```python
from build123d import *

# Parameters (mm, degrees)
SKETCH2_W           = 25
SKETCH2_H           = 62.5
SKETCH2_H_2         = 25
SKETCH2_W_2         = 62.5
BOSS_EXTRUDE3_DEPTH = 20
FILLET1_R           = 10
FILLET2_R           = 10
FILLET3_R           = 10
FILLET4_R           = 10
FILLET5_RADIUS      = 12.5
FILLET5_LENGTH      = 20
FILLET6_RADIUS      = 12.5
FILLET6_LENGTH      = 20
FILLET7_RADIUS      = 12.5
FILLET7_LENGTH      = 20
FILLET8_RADIUS      = 12.5
FILLET8_LENGTH      = 20
SKETCH4_R           = 2.5
CUT_EXTRUDE2_DEPTH  = 25
SKETCH5_R           = 37.5
BOSS_EXTRUDE4_DEPTH = 20
SKETCH7_R           = 2.5
CUT_EXTRUDE3_DEPTH  = 25
FILLET9_R           = 8


with BuildPart() as part:
    # Sketch2 → Boss-Extrude3 (new body)
    with BuildSketch(Plane(origin=(0, 0, 0), x_dir=(1, 0, 0), z_dir=(0, 1, 0))):
        with Locations((0, -43.75)):
            Rectangle(SKETCH2_W, SKETCH2_H)
        Rectangle(SKETCH2_W, SKETCH2_H_2)
        with Locations((0, 43.75)):
            Rectangle(SKETCH2_W, SKETCH2_H)
        with Locations((-43.75, 0)):
            Rectangle(SKETCH2_W_2, SKETCH2_H_2)
        with Locations((43.75, 0)):
            Rectangle(SKETCH2_W_2, SKETCH2_H_2)
    extrude(amount=BOSS_EXTRUDE3_DEPTH)

    # Fillet1
    fillet1_edges = [part.edges().sort_by_distance(p)[0] for p in [
        (-12.5, 10, 12.5),
    ]]
    fillet(fillet1_edges, radius=FILLET1_R)

    # Fillet2
    fillet2_edges = [part.edges().sort_by_distance(p)[0] for p in [
        (12.5, 10, 12.5),
    ]]
    fillet(fillet2_edges, radius=FILLET2_R)

    # Fillet3
    fillet3_edges = [part.edges().sort_by_distance(p)[0] for p in [
        (-12.5, 10, -12.5),
    ]]
    fillet(fillet3_edges, radius=FILLET3_R)

    # Fillet4
    fillet4_edges = [part.edges().sort_by_distance(p)[0] for p in [
        (12.5, 10, -12.5),
    ]]
    fillet(fillet4_edges, radius=FILLET4_R)

    # Fillet5: full round fillet: the end face becomes a half cylinder, R = half its width
    fillet5_face = Plane((75, 10, 0), x_dir=(0, 1, 0), z_dir=(1, 0, 0))  # on the end face: x along it, z out of the body
    fillet5_slab = fillet5_face.offset(-FILLET5_RADIUS / 2) * Box(FILLET5_LENGTH, 2 * FILLET5_RADIUS, FILLET5_RADIUS, mode=Mode.PRIVATE)  # the body's end, R deep
    fillet5_round = Plane((62.5, 10, 0), x_dir=(1, 0, 0), z_dir=(0, 1, 0)) * Cylinder(FILLET5_RADIUS, FILLET5_LENGTH, mode=Mode.PRIVATE)  # its axis R under the face
    add(fillet5_slab - fillet5_round, mode=Mode.SUBTRACT)

    # Fillet6: full round fillet: the end face becomes a half cylinder, R = half its width
    fillet6_face = Plane((0, 10, 75), x_dir=(0, 1, 0), z_dir=(0, 0, 1))  # on the end face: x along it, z out of the body
    fillet6_slab = fillet6_face.offset(-FILLET6_RADIUS / 2) * Box(FILLET6_LENGTH, 2 * FILLET6_RADIUS, FILLET6_RADIUS, mode=Mode.PRIVATE)  # the body's end, R deep
    fillet6_round = Plane((0, 10, 62.5), x_dir=(0, 0, 1), z_dir=(0, 1, 0)) * Cylinder(FILLET6_RADIUS, FILLET6_LENGTH, mode=Mode.PRIVATE)  # its axis R under the face
    add(fillet6_slab - fillet6_round, mode=Mode.SUBTRACT)

    # Fillet7: full round fillet: the end face becomes a half cylinder, R = half its width
    fillet7_face = Plane((-75, 10, 0), x_dir=(0, 1, 0), z_dir=(-1, 0, 0))  # on the end face: x along it, z out of the body
    fillet7_slab = fillet7_face.offset(-FILLET7_RADIUS / 2) * Box(FILLET7_LENGTH, 2 * FILLET7_RADIUS, FILLET7_RADIUS, mode=Mode.PRIVATE)  # the body's end, R deep
    fillet7_round = Plane((-62.5, 10, 0), x_dir=(-1, 0, 0), z_dir=(0, 1, 0)) * Cylinder(FILLET7_RADIUS, FILLET7_LENGTH, mode=Mode.PRIVATE)  # its axis R under the face
    add(fillet7_slab - fillet7_round, mode=Mode.SUBTRACT)

    # Fillet8: full round fillet: the end face becomes a half cylinder, R = half its width
    fillet8_face = Plane((0, 10, -75), x_dir=(0, 1, 0), z_dir=(0, 0, -1))  # on the end face: x along it, z out of the body
    fillet8_slab = fillet8_face.offset(-FILLET8_RADIUS / 2) * Box(FILLET8_LENGTH, 2 * FILLET8_RADIUS, FILLET8_RADIUS, mode=Mode.PRIVATE)  # the body's end, R deep
    fillet8_round = Plane((0, 10, -62.5), x_dir=(0, 0, -1), z_dir=(0, 1, 0)) * Cylinder(FILLET8_RADIUS, FILLET8_LENGTH, mode=Mode.PRIVATE)  # its axis R under the face
    add(fillet8_slab - fillet8_round, mode=Mode.SUBTRACT)

    # Sketch4 → Cut-Extrude2 (cut)
    with BuildSketch(Plane(origin=(0, 20, 0), x_dir=(1, 0, 0), z_dir=(0, 1, 0))):
        with Locations(Location((64, 0, 0), (0, 0, 270))):
            Circle(SKETCH4_R)
        with Locations(Location((0, -64, 0), (0, 0, 270))):
            Circle(SKETCH4_R)
        with Locations(Location((-64, 0, 0), (0, 0, 270))):
            Circle(SKETCH4_R)
        with Locations(Location((0, 64, 0), (0, 0, 270))):
            Circle(SKETCH4_R)
    extrude(amount=-CUT_EXTRUDE2_DEPTH, mode=Mode.SUBTRACT)

    # Sketch5 → Boss-Extrude4 (add)
    with BuildSketch(Plane(origin=(0, 20, 0), x_dir=(1, 0, 0), z_dir=(0, 1, 0))):
        Circle(SKETCH5_R)
    extrude(amount=-BOSS_EXTRUDE4_DEPTH)

    # Sketch7 → Cut-Extrude3 (cut)
    with BuildSketch(Plane(origin=(0, 20, 0), x_dir=(1, 0, 0), z_dir=(0, 1, 0))):
        with Locations(Location((0, 33, 0), (0, 0, 270))):
            Circle(SKETCH7_R)
        with Locations(Location((33, 0, 0), (0, 0, 270))):
            Circle(SKETCH7_R)
        with Locations(Location((0, -33, 0), (0, 0, 270))):
            Circle(SKETCH7_R)
        with Locations(Location((-33, 0, 0), (0, 0, 270))):
            Circle(SKETCH7_R)
    extrude(amount=-CUT_EXTRUDE3_DEPTH, mode=Mode.SUBTRACT)

    # Fillet9
    fillet9_edges = [part.edges().sort_by_distance(p)[0] for p in [
        (12.5, 10, 35.355339059),
        (35.355339059, 10, 12.5),
        (35.355339059, 10, -12.5),
        (12.5, 10, -35.355339059),
        (-35.355339059, 10, 12.5),
        (-12.5, 10, 35.355339059),
        (-12.5, 10, -35.355339059),
        (-35.355339059, 10, -12.5),
    ]]
    fillet(fillet9_edges, radius=FILLET9_R)


solid = part.part
```
The listing builds one solid part. Answer for the finished solid, in the listing's coordinates (mm). A direction names the side the tool comes from. Give positions to 0.01 mm unless a question says otherwise; leave off trailing zeros. Order: outer loops, then holes, each group sorted by start corner. A loop starts at its lowest first (then second) coordinate and runs counter-clockwise, first axis right, second up. Notation, with made-up numbers: (-16.5, 45) -> (8.5, 45) arc R25 cw to (8.5, 67) -> close; hole circle Ø9 at (-36.75, 66). An arc over 180 degrees is marked (long way). Write each question's results on one line, items separated by ' | '.
Q1. Each of these flat-tipped pins is pushed along its axis until it touches: P1, Ø1.5, axis at y = 12, z = -57, coming from the +X side; P2, Ø4, axis at y = 7, z = -40.5, coming from the +X side; P3, Ø10, axis at y = 6, z = 44, coming from the +X side; P4, Ø4.5, axis at x = 0, z = -33, coming from the -Y side. Where does it stop, or does it pass through?
Checked values:
P1: stops at x = 12.5 | P2: stops at x = 12.79 | P3: stops at x = 12.67 | P4: passes through
Q2. Which of the six approach directions +Z, -Z, +X, -X, +Y, -Y give full straight-line access (tool end or side, diameter ignored) to faces 1 (the face through (-0.96, 10.14, 35.31)), 2 (the face through (-12.5, 10, 51)), 3 (the face through (51, 10, -12.5))?
Checked values:
face 1: +Y, -Y | face 2: +Z, -X, +Y, -Y | face 3: -Z, +X, +Y, -Y
Q3. The part is cut by section C-C, the plane z = 59. Give the vertices of the cut face in (x, y), and give its area (3 significant figures).
Checked values:
outline: (-12.5, 0) -> (12.5, 0) -> (12.5, 20) -> (-12.5, 20) -> close | area: 500 mm^2
Q4. Straight lines are drawn through the part: probe 1 along X at (y, z) = (8.75, 0); probe 2 along X at (y, z) = (11, 1); probe 3 along X at (y, z) = (13.5, -64). For each, find the intervals that lie inside material, in ascending order. Write a range as from..to.
Checked values:
probe 1: x = -75..-66.5, -61.5..-35.5, -30.5..30.5, 35.5..61.5, 66.5..75 | probe 2: x = -74.96..-66.29, -61.71..-35.29, -30.71..30.71, 35.29..61.71, 66.29..74.96 | probe 3: x = -12.41..-2.5, 2.5..12.41
Q5. The part is cut by section A-A, the plane y = 11.5. State how many separate pieces and enclosed holes the cut face has, and give its area (3 significant figures).
Checked values:
separate pieces: 1 | enclosed holes: 8 | area: 7,850 mm^2
Q6. The part is cut by section B-B, the plane z = 0. Give the vertices of the cut face in (x, y).
Checked values:
outline: (-75, 0) -> (-66.5, 0) -> (-66.5, 20) -> (-75, 20) -> close; (-61.5, 0) -> (-35.5, 0) -> (-35.5, 20) -> (-61.5, 20) -> close; (-30.5, 0) -> (30.5, 0) -> (30.5, 20) -> (-30.5, 20) -> close; (35.5, 0) -> (61.5, 0) -> (61.5, 20) -> (35.5, 20) -> close; (66.5, 0) -> (75, 0) -> (75, 20) -> (66.5, 20) -> close
Q7. The part is cut by section D-D, the plane x = 48.5. Give the vertices of the cut face in (y, z).
Checked values:
outline: (0, -12.5) -> (20, -12.5) -> (20, 12.5) -> (0, 12.5) -> close
Q8. Determine the mould class of faces 4 (the face through (12.5, 10, 52)), 5 (the face through (0.751, 10.14, 66.385)), 6 (the face through (51, 10, 12.5)) for opening direction Z: pulls with the +Z half, pulls with the -Z half, needs draft (parallel to the pull), parting line crosses it, or undercut.
Checked values:
face 4: needs draft | face 5: undercut | face 6: pulls with the +Z half
